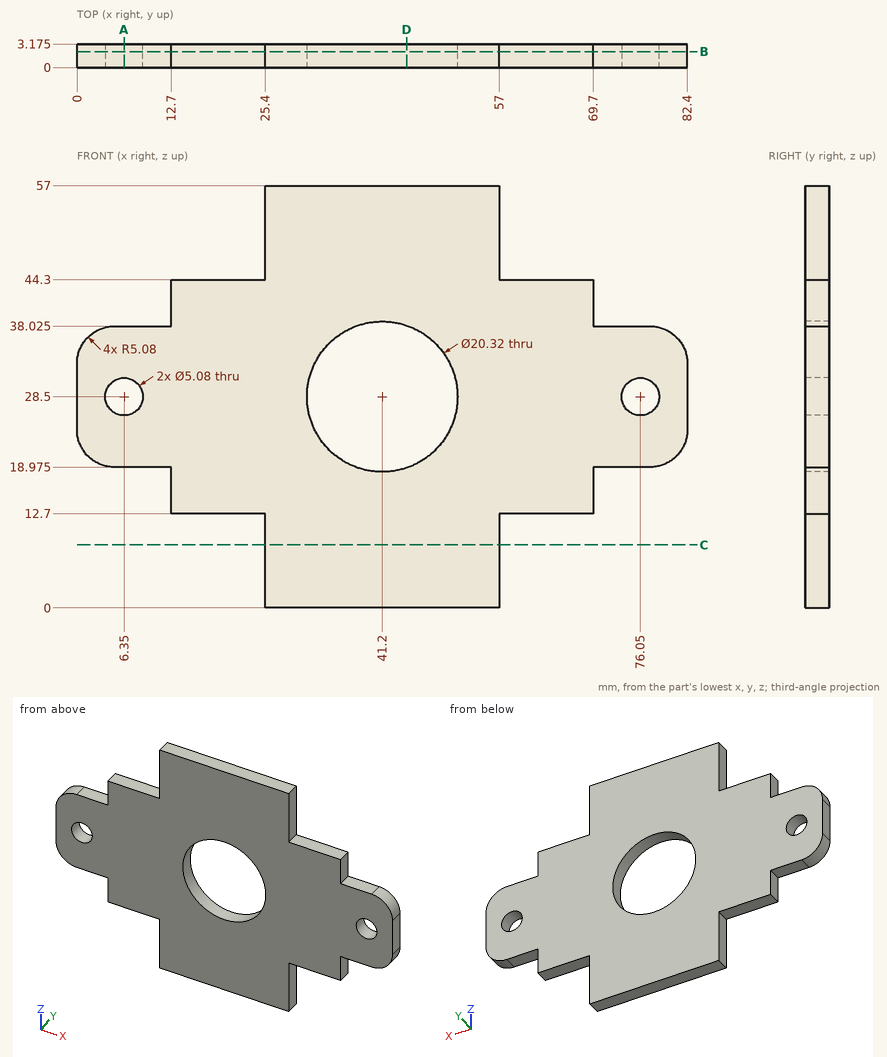
Design review of the part shown in the three views and the two pictorial views. Dimensions are in mm from the part's minimum x, y and z. Give positions to 0.01 mm unless a question says otherwise; leave off trailing zeros. Loops run counter-clockwise (first coordinate to the right, second up) from the corner with the lowest first, then second, coordinate; pieces in that order, holes last. Notation, with made-up numbers: M -38,-29 L 4,-29 A21 cw 4,-24 Z; hole C 31,-7.5 d3. An arc over 180 degrees is marked long. Answer as a JSON object with one key per item and string values. Group by question number.
Q1. Add section C-C on z = 8.5. Give the boundary of the cut face in (x, y) (3 decimals), and give its area (3 significant figures).
Q2. For probe 1 along X at (y, z) = (0.75, 28.5); probe 2 along Z at (x, y) = (6.35, 2.25) (3 decimals); probe 3 along X at (y, z) = (1.2, 27), list the stretches that pass through material, from the lowest coordinate up. Write a range as [from, to].
Q3. Add section B-B on y = 2.15. Give the boundary of the cut face in (x, z) (3 decimals).
Q4. Add section D-D on x = 44.5. Give the boundary of the cut face in (y, z) (3 decimals), and give its area (3 significant figures).
Q5. Add section A-A on x = 6.35. Give the boundary of the cut face in (y, z) (3 decimals).
Q6. Insertion check: P1, Ø1, axis at y = 2, z = 16.5, coming from the -X side; P2, Ø8, axis at x = 39, z = 18, coming from the -Y side; P3, Ø1.6, axis at y = 1, z = 15.5, coming from the +X side; P4, Ø1, axis at y = 1, z = 52.5, coming from the +X side. Each pin has a flat end and moves straight along its axis. Give the tip position at first contact, or say it passes through.
Checked values:
{
 "1": {"outline": "M 25.4,0 L 57,0 L 57,3.175 L 25.4,3.175 Z", "area": "100 mm²"},
 "2": {"probe 1": "[0, 3.81], [8.89, 31.04], [51.36, 73.51], [78.59, 82.4]", "probe 2": "[18.975, 25.96], [31.04, 38.025]", "probe 3": "[0, 4.3], [8.4, 31.15], [51.25, 74], [78.1, 82.4]"},
 "3": {"outline": "M 0,24.055 A5.08 ccw 5.08,18.975 L 12.7,18.975 L 12.7,12.7 L 25.4,12.7 L 25.4,0 L 57,0 L 57,12.7 L 69.7,12.7 L 69.7,18.975 L 77.32,18.975 A5.08 ccw 82.4,24.055 L 82.4,32.945 A5.08 ccw 77.32,38.025 L 69.7,38.025 L 69.7,44.3 L 57,44.3 L 57,57 L 25.4,57 L 25.4,44.3 L 12.7,44.3 L 12.7,38.025 L 5.08,38.025 A5.08 ccw 0,32.945 Z; hole C 6.35,28.5 d5.08; hole C 41.2,28.5 d20.32; hole C 76.05,28.5 d5.08"},
 "4": {"outline": "M 0,0 L 3.175,0 L 3.175,18.891 L 0,18.891 Z; M 0,38.109 L 3.175,38.109 L 3.175,57 L 0,57 Z", "area": "120 mm²"},
 "5": {"outline": "M 0,18.975 L 3.175,18.975 L 3.175,25.96 L 0,25.96 Z; M 0,31.04 L 3.175,31.04 L 3.175,38.025 L 0,38.025 Z"},
 "6": {"P1": "x = 12.7", "P2": "y = 0", "P3": "x = 69.7", "P4": "x = 57"}
}
